Build history of the part. All positions in model axes, mm. Round coordinates to 2 decimals unless told otherwise and drop trailing zeros. Write each loop counter-clockwise with the first axis right and the second up, starting at its lowest first coordinate (ties: lowest second). Pieces come first, ordered by that corner, then holes. Notation, with made-up numbers: (-29, 51.25) -> (-10, 51.25) arc R6 cw to (-10, 62.25) -> close; hole circle Ø8 at (14, 47). An arc over 180 degrees is marked (long way). One line per question, with ' | ' between items.
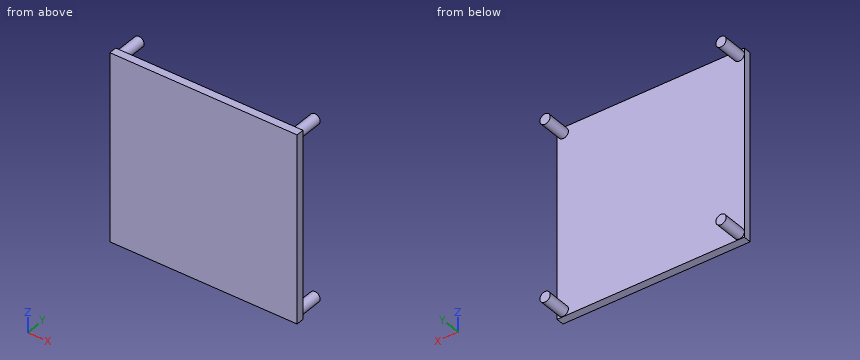
Autodesk Inventor part; units mm, degrees
ref_plane "YZ Plane" through (0, 0, 0) normal (1, 0, 0) x (0, 1, 0)
ref_plane "XZ Plane" through (0, 0, 0) normal (0, 1, 0) x (-1, 0, 0)
ref_plane "XY Plane" through (0, 0, 0) normal (0, 0, 1) x (1, 0, 0)
sketch "Sketch1" plane through (0, 0, 0) normal (0, 1, 0) x (-1, 0, 0)
  line L0 (19, 19) -> (-19, 19)
  line L1 (-19, 19) -> (-19, -19)
  line L2 (-19, -19) -> (19, -19)
  line L3 (19, -19) -> (19, 19)
  dimension "d0" = 38
  dimension "d1" = 38
extrude "Extrusion1" add sketch "Sketch1" along normal blind 1.6
sketch "Sketch2" plane through (0, 1.6, 0) normal (0, 1, 0) x (1, 0, 0)
  line L0 (19, -19) -> (19, 19)
  circle A0 centre (17.7429, 17.8888) radius 1.05
  circle A1 centre (17.7429, -17.8399) radius 1.05
  circle A2 centre (-17.9859, -17.8399) radius 1.05
  circle A3 centre (-17.9859, 17.8888) radius 1.05
  point P0 (0, 0)
  dimension "d7" = 2.1
  dimension "d8" = 2.1
  dimension "d9" = 2.1
  dimension "d10" = 2.1
extrude "Extrusion2" add sketch "Sketch2" along normal blind 4.95
sketch "Sketch3" plane through (0, 1.6, 0) normal (0, 1, 0) x (1, 0, 0)
  point P0 (0, 0)
properties part number "Camera Bottom"
(1) Drop flat-ended pins along their axis: pin 1 (2 mm diameter, centred on x = 10, z = -11, fed in from +Y); pin 2 (0.5 mm diameter, centred on y = 0.5, z = 7, fed in from -X); pin 3 (3 mm diameter, centred on y = 4, z = -14, fed in from -X). Give the stop position or say it passes through.
Calculated:
pin 1: y = 1.6 | pin 2: x = -19 | pin 3: through
(2) Slice it at C-C (y = 5). Write the cut outline in (x, z).
Calculated:
outline: circle Ø2.1 at (-17.99, -17.89); circle Ø2.1 at (-17.99, 17.84); circle Ø2.1 at (17.74, -17.89); circle Ø2.1 at (17.74, 17.84)
(3) Wall check: line 1 (Y direction, x = 14, z = -9); line 2 (X direction, y = 1.5, z = 15). Give the ranges that are in metal, low to high. Write a range as from..to.
Calculated:
line 1: 0..1.6 | line 2: -19..19
(4) Slice it at B-B (z = 4.5). Write the cut outline in (x, y).
Calculated:
outline: (-19, 0) -> (19, 0) -> (19, 1.6) -> (-19, 1.6) -> close
(5) Slice it at A-A (x = -7). Write the cut outline in (y, z), then the cut area to 3 significant figures.
Calculated:
outline: (0, -19) -> (1.6, -19) -> (1.6, 19) -> (0, 19) -> close | area: 60.8 mm2
